Verification items for the finished model (mm, model axes). Face numbers are marked on the shaded views. A direction names the side the tool comes from. Round coordinates to 2 decimals unless told otherwise and drop trailing zeros. Order: outer loops, then holes, each group sorted by start corner. A loop starts at its lowest first (then second) coordinate and runs counter-clockwise, first axis right, second up. Notation, with made-up numbers: M 72,39.25 L 91,39.25 A21 ccw 91,65.25 Z; hole C 1.25,16.25 d6. An arc over 180 degrees is marked long. Use one line per item in the form item = value. Start each with the question number.
Item 1: Release check for a two-part mould opening along Y. For the marked faces 3, 4 and 5 record: +Y half, -Y half, draft (parallel to the pull), parting line (faces both ways), or undercut.
Item 2: Go/stop test with flat-tipped pins: pin 1 Ø4 at (x, z) = (-30.5, 12) entering from -Y; pin 2 Ø10 at (x, y) = (-9.5, -6) entering from +Z; pin 3 Ø1 at (y, z) = (-11, 2) entering from +X. Record where each tip stops, or that it passes through.
Item 3: Cross-section at A-A on x = 0. Enter the section's corners in (y, z) (3 decimals), then the cut area to 3 significant figures.
Item 4: Tool access check on the marked faces 1 and 2. Record the directions out of +Z, -Z, +X, -X, +Y, -Y that give a thin tool (end or side, any length) a straight path to the whole face; none if there is none.
Item 5: Thickness scan on probe 1 along Z at (x, y) = (3.5, -1); probe 2 along Y at (x, z) = (23.5, 7.25); probe 3 along Y at (x, z) = (33, 8.5). Record the ranges inside material, lowest first. Write a range as [from, to].
Item 6: Cross-section at C-C on y = -17. Enter the section's corners in (x, z).
Item 7: Cross-section at D-D on z = 13.75. Enter the section's corners in (x, y) (3 decimals), then the cut area to 3 significant figures.
from build123d import *

# Parameters (mm, degrees)
F2_R     = 2.54
F3_DEPTH = 25.4
F4_R     = 2.54
F5_DEPTH = 25.4


with BuildPart() as f1:
    # F0 (on Right) → F1 (revolve)
    with BuildSketch(Plane.YZ):
        Polygon((0, 6.35), (0, 0), (38.1, 0), (38.1, 19.05), (31.75, 19.05), (31.75, 6.35), align=None)
    revolve(axis=Axis((0, 0, 3.175), (0, 0, -1)))

    # F2 (on face) → F3 (cut)
    with BuildSketch(Plane.XY.offset(6.35)):
        Circle(F2_R)
    extrude(amount=-F3_DEPTH, mode=Mode.SUBTRACT)

    # F4 (on face) → F5 (cut)
    with BuildSketch(Plane.XY.offset(19.05)):
        with Locations((0, 34.925)):
            Circle(F4_R)
        with Locations((34.925, 0)):
            Circle(F4_R)
        with Locations((-34.925, 0)):
            Circle(F4_R)
        with Locations((0, -34.925)):
            Circle(F4_R)
    extrude(amount=-F5_DEPTH, mode=Mode.SUBTRACT)


solid = f1.part
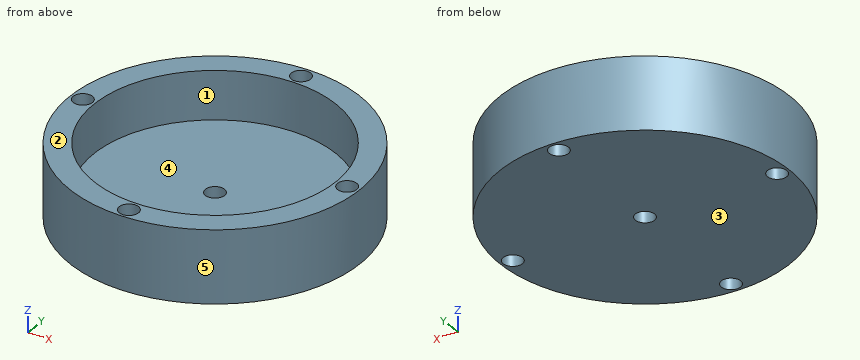
Output values:
q1.face_3 = draft
q1.face_4 = undercut
q1.face_5 = parting line
q2.pin_1 = -25.29
q2.pin_2 = 6.35
q2.pin_3 = 36.62
q3.outline = M -38.1,0 L -37.465,0 L -37.465,19.05 L -38.1,19.05 Z; M -32.385,0 L -2.54,0 L -2.54,6.35 L -31.75,6.35 L -31.75,19.05 L -32.385,19.05 Z; M 2.54,0 L 32.385,0 L 32.385,19.05 L 31.75,19.05 L 31.75,6.35 L 2.54,6.35 Z; M 37.465,0 L 38.1,0 L 38.1,19.05 L 37.465,19.05 Z
q3.area = 419 mm2
q4.face_1 = +Z
q4.face_2 = +Z, +X, -X, +Y, -Y
q5.probe_1 = [0, 6.35]
q5.probe_2 = [-29.99, -21.35], [21.35, 29.99]
q5.probe_3 = [-19.04, -1.66], [1.66, 19.04]
q6.outline = M -34.1,0 L 34.1,0 L 34.1,19.05 L 26.82,19.05 L 26.82,6.35 L -26.82,6.35 L -26.82,19.05 L -34.1,19.05 Z
q7.outline = C 0,0 d76.2; hole C -34.925,0 d5.08; hole C 0,0 d63.5; hole C 0,-34.925 d5.08; hole C 0,34.925 d5.08; hole C 34.925,0 d5.08
q7.area = 1,310 mm2
